```python
from build123d import *

# Parameters (mm, degrees)
EXTRUDE_1_DEPTH                 = 5
SKETCH_3_W                      = 50
SKETCH_3_H                      = 5
SKETCH_7_W                      = 100
SKETCH_7_H                      = 5
CUT_EXTRUDE_1_DEPTH             = 324.341924284
CUT_EXTRUDE_1_DEPTH_BACK        = 324.341924284
SKETCH_8_R                      = 2
SKETCH_6_W                      = 5
SKETCH_6_H                      = 50
SKETCH_9_R                      = 2
CUT_EXTRUDE_2_DEPTH             = 50
SKETCH_10_R                     = 6
CUT_EXTRUDE_3_DEPTH             = 105
CUT_EXTRUDE_4_REACH             = 369.526
SKETCH_11_R                     = 2
CUT_EXTRUDE_4_DIRECTION_2_REACH = 369.526
SKETCH_12_R                     = 6
CUT_EXTRUDE_5_DEPTH             = 210
SKETCH_13_R                     = 6
CUT_EXTRUDE_6_DEPTH             = 36
SCALE_1_SCALE                   = 0.5
CUT_EXTRUDE_8_DEPTH             = 10


with BuildPart() as part:
    # 草图1 → 凸台-拉伸1 (new body)
    with BuildSketch(Plane.XY):
        Polygon((-200, 0), (-100, 200), (100, 200), (200, 0), align=None)
    extrude(amount=EXTRUDE_1_DEPTH)

    # 草图3 → 旋转5 (revolve)
    with BuildSketch(Plane.XZ):
        with Locations((130, 2.5)):
            Rectangle(SKETCH_3_W, SKETCH_3_H)
        with Locations((-130, 2.5)):
            Rectangle(SKETCH_3_W, SKETCH_3_H)
    revolve(axis=Axis((-155, 0, 0), (1, 0, 0)))

    # 草图7 → 旋转1 (revolve)
    with BuildSketch(Plane(origin=(0, 0, 0), x_dir=(-1, 0, 0), z_dir=(0, 0, -1))):
        with Locations((0, 197.5)):
            Rectangle(SKETCH_7_W, SKETCH_7_H)
    revolve(axis=Axis((50, 200, 0), (-1, 0, 0)))

    # 草图8 → 切除-拉伸1 (cut, two sides: drawn at the far end of the back side and taken through both)
    with BuildSketch(Plane(origin=(50, 0, 0), x_dir=(0, 0, -1), z_dir=(1, 0, 0)).offset(-CUT_EXTRUDE_1_DEPTH_BACK)):
        with Locations(Location((0, 200, 0), (0, 0, 270))):
            Circle(SKETCH_8_R)
    extrude(amount=CUT_EXTRUDE_1_DEPTH + CUT_EXTRUDE_1_DEPTH_BACK, mode=Mode.SUBTRACT)

    # 草图6 → 旋转4 (revolve)
    with BuildSketch(Plane(origin=(-160, 80, 0), x_dir=(0, 0, 1), z_dir=(-0.8944271909999159, 0.44721359549995815, 0))):
        with Locations((2.5, -27.639320225)):
            Rectangle(SKETCH_6_W, SKETCH_6_H)
    revolve_4 = revolve(axis=Axis((-161.180339887, 77.639320225, 0), (-0.447213595499958, -0.894427190999916, 0)))

    # 草图9 → 切除-拉伸2 (cut)
    with BuildSketch(Plane(origin=(-23.541019662, -47.082039325, 0), x_dir=(0.8944271909999156, -0.4472135954999583, 0), z_dir=(-0.4472135954999583, -0.8944271909999156, 0))):
        with Locations((-178.8854382, 0)):
            Circle(SKETCH_9_R)
    cut_extrude_2 = extrude(amount=-CUT_EXTRUDE_2_DEPTH, mode=Mode.SUBTRACT)

    # 草图10 → 切除-拉伸3 (cut)
    with BuildSketch(Plane(origin=(-1.180339887, -2.360679775, 0), x_dir=(0.8944271909999156, -0.4472135954999583, 0), z_dir=(0.4472135954999583, 0.8944271909999156, 0))):
        with Locations((-178.8854382, 0)):
            Circle(SKETCH_10_R)
    cut_extrude_3 = extrude(amount=CUT_EXTRUDE_3_DEPTH, mode=Mode.SUBTRACT)

    # 切除-拉伸4: up to this face of the body (flat: up to its plane)
    cut_extrude_4_end = Plane(part.part.faces().sort_by_distance((155, -0.707355303, -0.707355303))[0])
    # 草图11 → 切除-拉伸4 (cut, up to the picked face)
    with BuildSketch(Plane(origin=(-105, 0, 0), x_dir=(0, 0, -1), z_dir=(1, 0, 0)), mode=Mode.PRIVATE) as cut_extrude_4_sk1:
        with Locations(Location((0, 0, 0), (0, 0, 180))):
            Circle(SKETCH_11_R)
    cut_extrude_4_tool1 = split(extrude(cut_extrude_4_sk1.sketch, amount=CUT_EXTRUDE_4_REACH, mode=Mode.PRIVATE), bisect_by=cut_extrude_4_end, keep=Keep.BOTH, mode=Mode.PRIVATE)
    add(cut_extrude_4_tool1.solids().sort_by(Axis((-105, 0, 0), (1, 0, 0)))[0], mode=Mode.SUBTRACT)

    # 切除-拉伸4 direction 2: up to this face of the body (flat: up to its plane)
    cut_extrude_4_direction_2_end = Plane(part.part.faces().sort_by_distance((-155, -0.707355303, -0.707355303))[0])
    # 草图11 → 切除-拉伸4 direction 2 (cut, up to the picked face)
    with BuildSketch(Plane(origin=(-105, 0, 0), x_dir=(0, 0, -1), z_dir=(1, 0, 0)), mode=Mode.PRIVATE) as cut_extrude_4_direction_2_sk1:
        with Locations(Location((0, 0, 0), (0, 0, 180))):
            Circle(SKETCH_11_R)
    cut_extrude_4_direction_2_tool1 = split(extrude(cut_extrude_4_direction_2_sk1.sketch, amount=-CUT_EXTRUDE_4_DIRECTION_2_REACH, mode=Mode.PRIVATE), bisect_by=cut_extrude_4_direction_2_end, keep=Keep.BOTH, mode=Mode.PRIVATE)
    add(cut_extrude_4_direction_2_tool1.solids().sort_by(Axis((-105, 0, 0), (-1, 0, 0)))[0], mode=Mode.SUBTRACT)

    # 镜向1: 旋转4, 切除-拉伸2, 切除-拉伸3 across plane
    add(revolve_4.mirror(Plane(origin=(0, 0, 0), x_dir=(0, 0, 1), z_dir=(1, 0, 0))))
    add(cut_extrude_2.mirror(Plane(origin=(0, 0, 0), x_dir=(0, 0, 1), z_dir=(1, 0, 0))), mode=Mode.SUBTRACT)
    add(cut_extrude_3.mirror(Plane(origin=(0, 0, 0), x_dir=(0, 0, 1), z_dir=(1, 0, 0))), mode=Mode.SUBTRACT)

    # 草图12 → 切除-拉伸5 (cut)
    with BuildSketch(Plane.ZY.offset(-105)):
        Circle(SKETCH_12_R)
    extrude(amount=CUT_EXTRUDE_5_DEPTH, mode=Mode.SUBTRACT)

    # 草图13 → 切除-拉伸6 (cut)
    with BuildSketch(Plane.ZY.offset(50)):
        with Locations((0, 200)):
            Circle(SKETCH_13_R)
    cut_extrude_6 = extrude(amount=CUT_EXTRUDE_6_DEPTH, mode=Mode.SUBTRACT)

    # 镜向2: 切除-拉伸6 across plane
    add(cut_extrude_6.mirror(Plane(origin=(0, 0, 0), x_dir=(0, 0, 1), z_dir=(1, 0, 0))), mode=Mode.SUBTRACT)


with BuildPart() as part_1:
    # 缩放比例1: scaled about (0, 0, 0)
    add(part.part.scale(SCALE_1_SCALE))

    # 草图18 → 切除-拉伸8 (cut)
    with BuildSketch(Plane.XY.offset(2.5)):
        Polygon((27.5, 98.341687605), (27.5, 88.25), (17.5, 88.25), (17.5, 77.25), (9.5, 77.25), (9.5, 82.25), (-7.5, 82.25), (-7.5, 102.5), (25, 102.5), (25, 98.341687605), align=None)
    extrude(amount=-CUT_EXTRUDE_8_DEPTH, mode=Mode.SUBTRACT)


solid = part_1.part
```
Input: part model. Units: mm. Frame: model coordinates. A direction names the side the tool comes from. Give positions to 0.01 mm unless a question says otherwise; leave off trailing zeros. Order: outer loops, then holes, each group sorted by start corner. A loop starts at its lowest first (then second) coordinate and runs counter-clockwise, first axis right, second up. Notation, with made-up numbers: M 19.5,9 L 46.5,9 A23 ccw 46.5,19 Z; hole C -2.5,63 d1. An arc over 180 degrees is marked long. Return JSON: item names as keys, results as strings.
1) Section query A-A on x = -32. Output: boundary loops of the cut face in (y, z).
Taken from the geometry:
{"outline": "M 1.66,2.5 A3 cw 3,0 L 97,0 A3 cw 98.34,2.5 Z"}
2) Access query for faces 1 (the face through (96, 8, 1)), 2 (the face through (-92.299, 16.723, -1.076)), 3 (the face through (-52.5, 1, 1)), 4 (the face through (80.401, 38.725, 1.146)). Directions: +Z, -Z, +X, -X, +Y, -Y. A direction counts if a zero-diameter tool reaches every point of the face in a straight line with its end or side. Return the directions, or none.
Taken from the geometry:
{"face 1": "+Z, -Z, +X", "face 2": "-Z, -X", "face 3": "-Z, -Y", "face 4": "-Z, +Y"}
3) Contact query for flat-ended pins moving along their axis: pin 1 (1 mm diameter, centred on x = -55, y = 26, fed in from -Z); pin 2 (1.2 mm diameter, centred on y = 80.5, z = 2, fed in from +X); pin 3 (0.8 mm diameter, centred on x = -83.5, z = 0.5, fed in from -Y); pin 4 (2 mm diameter, centred on y = 47.5, z = -2, fed in from -X). Output: stop coordinate, or through.
Taken from the geometry:
{"pin 1": "stops at z = 0", "pin 2": "stops at x = 58.06", "pin 3": "stops at y = 0", "pin 4": "passes through"}
4) Line query: L1, parallel to Z at x = -11.5, y = 76; L2, parallel to X at y = 28, z = 0.2; L3, parallel to X at y = 21, z = 0.7. Output: solid intervals per line, ascending. Write a range as [from, to].
Taken from the geometry:
{"L1": "z = [0, 2.5]", "L2": "x = [-88.79, -87.1], [-84.9, 84.9], [87.1, 88.79]", "L3": "x = [-92.18, -90.3], [-88.7, 88.7], [90.3, 92.18]"}
5) Mould query, pull axis X, two halves, no side actions, for faces 5 (the face through (-87.15, 27.93, 0.04)), 6 (the face through (65.175, -1.825, -1.709)), 7 (the face through (92.299, 16.723, -1.076)). Classes: released by +X, released by -X, zero draft, split by the parting line, or undercut.
Taken from the geometry:
{"face 5": "undercut", "face 6": "zero draft", "face 7": "released by +X"}
